Design review of the part shown in the three views and the two pictorial views. Dimensions are in mm from the part's minimum x, y and z. Round coordinates to 2 decimals unless told otherwise and drop trailing zeros. Order: outer loops, then holes, each group sorted by start corner. A loop starts at its lowest first (then second) coordinate and runs counter-clockwise, first axis right, second up. Notation, with made-up numbers: (89, -24.5) - (120, -24.5) arc R24 ccw to (120, -6.5) - close; hole circle Ø8 at (37.25, -27). An arc over 180 degrees is marked (long way). One line per question, with ' | ' between items. Start each with the question number.
Item 1: Draft analysis for pull direction X (two halves, no side actions). For the marked faces 1, 2 and 3, state which applies: +X half, -X half, draft (parallel to the pull), parting line (faces both ways), or undercut.
Item 2: Add section C-C on z = 17. State the section outline as (x, y) points.
Item 3: Add section D-D on y = 9. State how many separate pieces and enclosed holes the cut face has.
Item 4: For L1, parallel to Z at x = 19.5, y = 8.75 (1 decimal); L2, parallel to Z at x = 18, y = 1.5 (1 decimal); L3, parallel to Z at x = 6.35, y = 8, list the stretches that pass through material, from the lowest coordinate up. Write a range as [from, to].
Item 5: Add section B-B on x = 20. State the section outline as (y, z) points, and give its area (3 significant figures).
Item 6: Add section A-A on x = 6.35. State the section outline as (y, z) points, and give its area (3 significant figures).
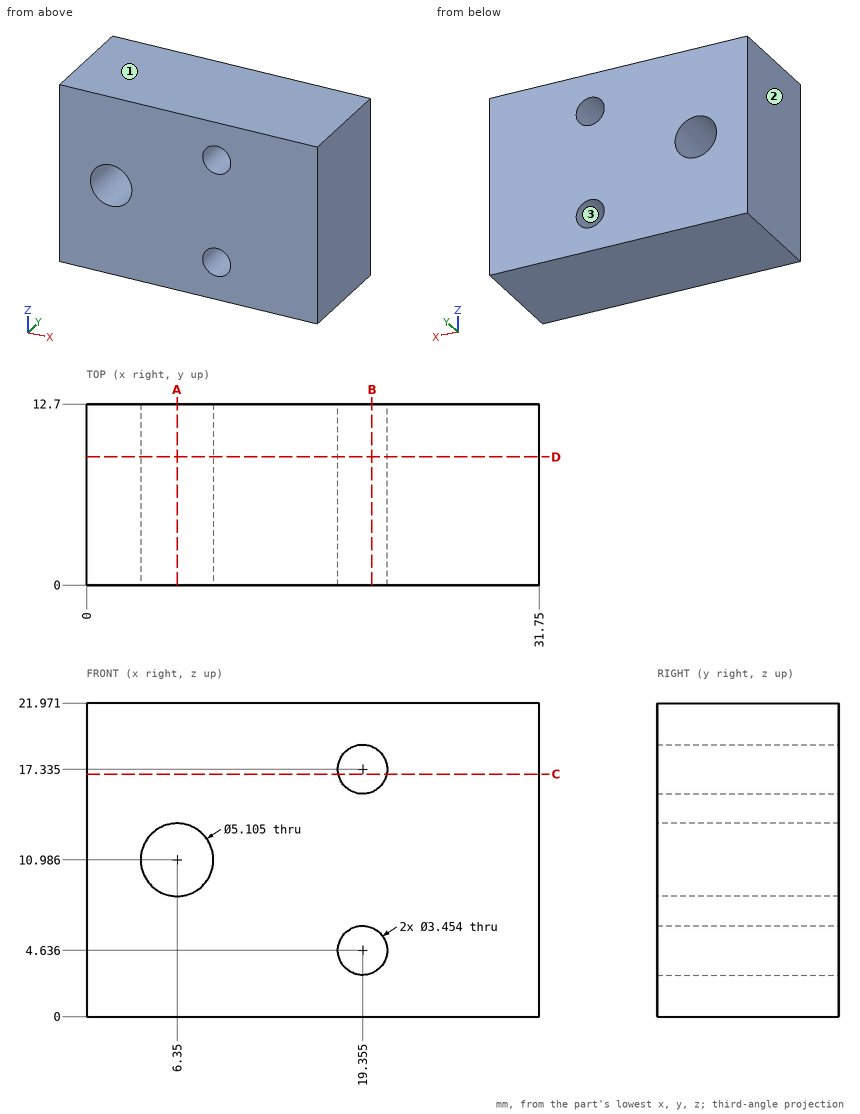
Determined:
1) face 1: draft | face 2: -X half | face 3: undercut
2) outline: (0, 0) - (17.66, 0) - (17.66, 12.7) - (0, 12.7) - close; (21.05, 0) - (31.75, 0) - (31.75, 12.7) - (21.05, 12.7) - close
3) separate pieces: 1 | enclosed holes: 3
4) L1: [0, 2.9], [6.4, 15.6], [19.1, 22] | L2: [0, 3.6], [5.7, 16.3], [18.4, 22] | L3: [0, 8.43], [13.54, 21.97]
5) outline: (0, 0) - (12.7, 0) - (12.7, 3.03) - (0, 3.03) - close; (0, 6.24) - (12.7, 6.24) - (12.7, 15.73) - (0, 15.73) - close; (0, 18.94) - (12.7, 18.94) - (12.7, 21.97) - (0, 21.97) - close | area: 198 mm2
6) outline: (0, 0) - (12.7, 0) - (12.7, 8.43) - (0, 8.43) - close; (0, 13.54) - (12.7, 13.54) - (12.7, 21.97) - (0, 21.97) - close | area: 214 mm2
